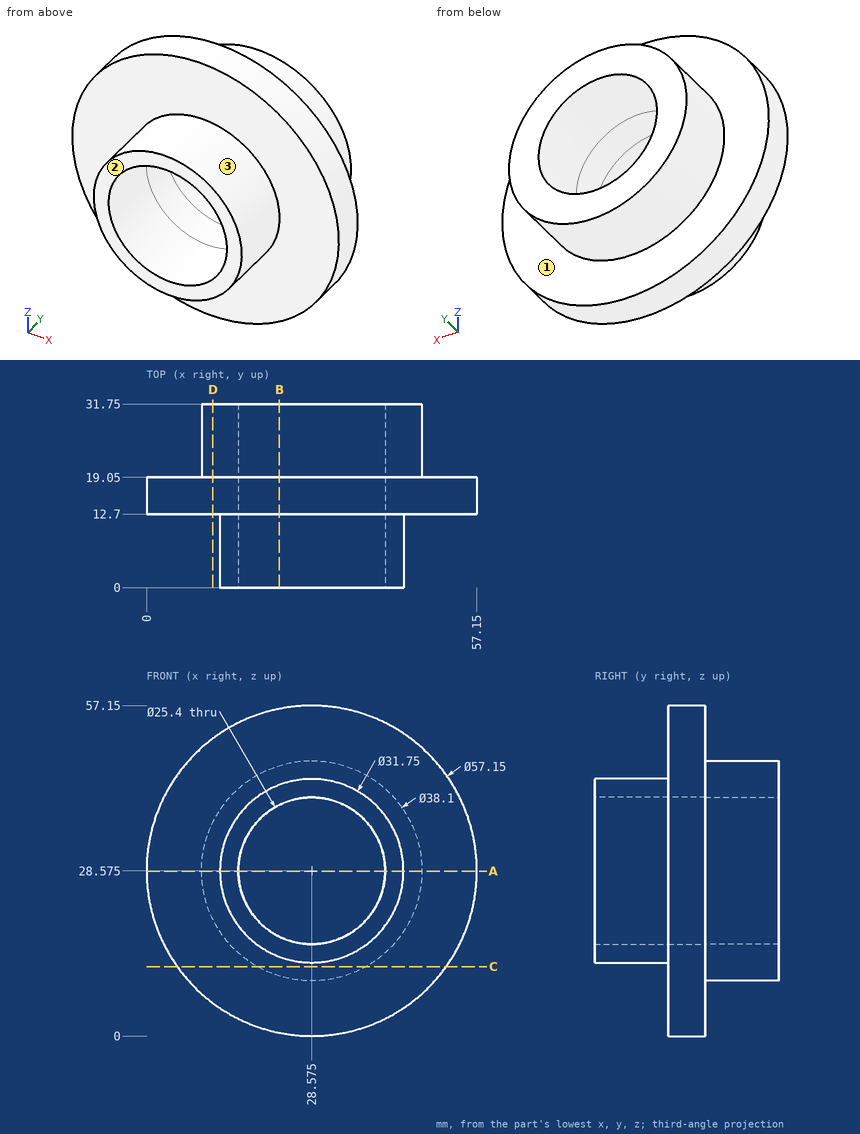
Geometry: see drawing. Coordinates: mm, zero at the bounding-box minimum. A direction names the side the tool comes from. Give positions to 0.01 mm unless a question says otherwise; leave off trailing zeros. Order: outer loops, then holes, each group sorted by start corner. A loop starts at its lowest first (then second) coordinate and runs counter-clockwise, first axis right, second up.
1. Set-up query: the marked faces 1, 2 and 3. Return all of +Z, -Z, +X, -X, +Y, -Y with unobstructed straight access to the full face (end or side cutting, diameter ignored); none if empty.
Computed:
face 1: +Y
face 2: +Z, -Z, +X, -X, -Y
face 3: -Y
2. Line query: probe 1 along Y at (x, z) = (52, 40); probe 2 along Z at (x, y) = (18, 4); probe 3 along X at (y, z) = (27.5, 40). Output: solid intervals per line, ascending.
Computed:
probe 1: y = 12.7 to 19.05
probe 2: z = 16.74 to 21.54, 35.61 to 40.41
probe 3: x = 13.33 to 23.03, 34.12 to 43.82
3. Cut plane B-B (x = 23). Return loops of the section in (y, z), and give its area (3 significant figures).
Computed:
outline: (0, 13.71) - (12.7, 13.71) - (12.7, 0.55) - (19.05, 0.55) - (19.05, 10.36) - (31.75, 10.36) - (31.75, 17.16) - (0, 17.16) - close; (0, 39.99) - (31.75, 39.99) - (31.75, 46.79) - (19.05, 46.79) - (19.05, 56.6) - (12.7, 56.6) - (12.7, 43.44) - (0, 43.44) - close
area: 472 mm2
4. Pin query (flat end, axial travel): pin 1 Ø12 at (y, z) = (10, 19) entering from +X; pin 2 Ø5 at (x, z) = (44.5, 41) entering from +Y; pin 3 Ø4 at (x, z) = (15.5, 9) entering from -Y; pin 4 Ø10 at (x, y) = (35, 28) entering from +Z. Return the tip coordinate at first contact, or that it passes through.
Computed:
pin 1: stops at x = 56.84
pin 2: stops at y = 31.75
pin 3: stops at y = 12.7
pin 4: stops at z = 47.57
5. Cut plane A-A (z = 28.5). Return loops of the section in (x, y).
Computed:
outline: (0, 12.7) - (12.7, 12.7) - (12.7, 0) - (15.88, 0) - (15.88, 31.75) - (9.53, 31.75) - (9.53, 19.05) - (0, 19.05) - close; (41.27, 0) - (44.45, 0) - (44.45, 12.7) - (57.15, 12.7) - (57.15, 19.05) - (47.62, 19.05) - (47.62, 31.75) - (41.27, 31.75) - close
6. Cut plane C-C (z = 12). Return loops of the section in (x, y).
Computed:
outline: (5.3, 12.7) - (51.85, 12.7) - (51.85, 19.05) - (37.96, 19.05) - (37.96, 31.75) - (19.19, 31.75) - (19.19, 19.05) - (5.3, 19.05) - close
7. Cut plane D-D (x = 11.5). Return loops of the section in (y, z).
Computed:
outline: (12.7, 5.66) - (19.05, 5.66) - (19.05, 20.13) - (31.75, 20.13) - (31.75, 37.02) - (19.05, 37.02) - (19.05, 51.49) - (12.7, 51.49) - close
